Here's how the part is built. I have some questions about the finished solid (model axes, mm). Face numbers are marked on the shaded views. A direction names the side the tool comes from. Round coordinates to 2 decimals unless told otherwise and drop trailing zeros. Write each loop counter-clockwise with the first axis right and the second up, starting at its lowest first coordinate (ties: lowest second). Pieces come first, ordered by that corner, then holes. Notation, with made-up numbers: (17.25, 31.25) - (28.25, 31.25) arc R31 ccw to (28.25, 61.25) - close; hole circle Ø8 at (41.5, -23.75). An arc over 180 degrees is marked (long way). One line per question, with ' | ' between items. Start each with the question number.
(1) Will these pins go through, and if not, where does the flat tip stop? pin 1 (11 mm diameter, centred on x = -95.5, y = -3.5, fed in from +Z); pin 2 (1.6 mm diameter, centred on y = -43.5, z = -120.5, fed in from +X); pin 3 (1 mm diameter, centred on y = -36, z = -56.5, fed in from -X).
(2) Imagine slicing it at C-C (y = -13.5). Write out the boundary of the cut face in (x, z).
(3) For the marked faces 1 and 2, which set-ups out of +Z, -Z, +X, -X, +Y, -Y let a thin tool reach every point of the face, with its end or its side?
(4) If I drill on L1, parallel to X at y = -44, z = -79; L2, parallel to X at y = -31, z = -190; L3, parallel to Y at x = -59.5, z = -171.5, over which ranges is the centre line in solid material (lowest first)?
(5) Imagine slicing it at D-D (x = -29). Write out the boundary of the cut face in (y, z).
(6) Imagine slicing it at A-A (x = -93). Write out the boundary of the cut face in (y, z).
(7) Thinking about a two-plate mould opening in X: for the marked faces 3 and 4, which applies, pulls with the +X half, pulls with the -X half, needs draft (parallel to the pull), parting line crosses it, or undercut?
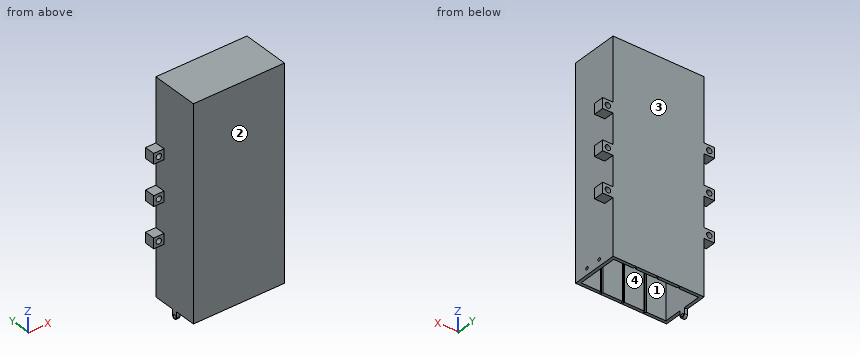
from build123d import *

# Parameters (mm, degrees)
SKETCH1_W           = 88
SKETCH1_H           = 46
SKETCH1_W_2         = 82
SKETCH1_H_2         = 40
BOSS_EXTRUDE1_DEPTH = 3
SKETCH3_W           = 88
SKETCH3_H           = 46
BOSS_EXTRUDE2_DEPTH = 200
SKETCH4_W           = 10
SKETCH4_H           = 10
BOSS_EXTRUDE3_DEPTH = 10
SKETCH7_R           = 2.6
CUT_EXTRUDE1_DEPTH  = 228.420315715
SKETCH8_W           = 3
SKETCH8_H           = 5
BOSS_EXTRUDE4_DEPTH = 8
FILLET1_RADIUS      = 2.5
FILLET1_LENGTH      = 3
SKETCH10_R          = 1.5
CUT_EXTRUDE3_DEPTH  = 10
SKETCH9_R           = 1.5
CUT_EXTRUDE4_DEPTH  = 10


with BuildPart() as part:
    # Sketch1 → Boss-Extrude1 (new body)
    # profile 1 of 2: a face of its own
    with BuildSketch(Plane.XY):
        with Locations((-44, -23)):
            Rectangle(SKETCH1_W, SKETCH1_H)
        with Locations((-44, -23)):
            Rectangle(SKETCH1_W_2, SKETCH1_H_2, mode=Mode.SUBTRACT)
    # profile 2 of 2: a face of its own
    with BuildSketch(Plane.XY):
        with Locations((-44, -23)):
            Rectangle(SKETCH1_W_2, SKETCH1_H_2)
    extrude(amount=BOSS_EXTRUDE1_DEPTH)

    # Sketch3 → Boss-Extrude2 (add)
    with BuildSketch(Plane(origin=(0, 0, 0), x_dir=(-1, 0, 0), z_dir=(0, 0, -1))):
        with Locations((44, -23)):
            Rectangle(SKETCH3_W, SKETCH3_H)
        Polygon((24, -3), (43, -3), (43, -1.5), (45, -1.5), (45, -3), (64, -3), (64, -1.5), (66, -1.5), (66, -3), (85, -3), (85, -43), (66, -43), (66, -44.5), (64, -44.5), (64, -43), (45, -43), (45, -44.5), (43, -44.5), (43, -43), (24, -43), (24, -44.5), (22, -44.5), (22, -43), (3, -43), (3, -3), (22, -3), (22, -1.5), (24, -1.5), align=None, mode=Mode.SUBTRACT)
    extrude(amount=BOSS_EXTRUDE2_DEPTH)

    # Sketch4 → Boss-Extrude3 (add)
    with BuildSketch(Plane(origin=(0, 0, 0), x_dir=(1, 0, 0), z_dir=(0, 1, 0))):
        with Locations((5, 141)):
            Rectangle(SKETCH4_W, SKETCH4_H)
        with Locations((5, 102)):
            Rectangle(SKETCH4_W, SKETCH4_H)
        with Locations((5, 63)):
            Rectangle(SKETCH4_W, SKETCH4_H)
        with Locations((-93, 141)):
            Rectangle(SKETCH4_W, SKETCH4_H)
        with Locations((-93, 102)):
            Rectangle(SKETCH4_W, SKETCH4_H)
        with Locations((-93, 63)):
            Rectangle(SKETCH4_W, SKETCH4_H)
    extrude(amount=-BOSS_EXTRUDE3_DEPTH)

    # Sketch7 → Cut-Extrude1 (cut, through all)
    with BuildSketch(Plane(origin=(0, 0, 0), x_dir=(1, 0, 0), z_dir=(0, 1, 0))):
        with Locations(Location((-93, 141, 0), (0, 0, 270))):
            Circle(SKETCH7_R)
        with Locations(Location((-93, 102, 0), (0, 0, 270))):
            Circle(SKETCH7_R)
        with Locations(Location((-93, 63, 0), (0, 0, 270))):
            Circle(SKETCH7_R)
        with Locations(Location((5, 141, 0), (0, 0, 270))):
            Circle(SKETCH7_R)
        with Locations(Location((5, 102, 0), (0, 0, 270))):
            Circle(SKETCH7_R)
        with Locations(Location((5, 63, 0), (0, 0, 270))):
            Circle(SKETCH7_R)
    extrude(amount=-CUT_EXTRUDE1_DEPTH, mode=Mode.SUBTRACT)

    # Sketch8 → Boss-Extrude4 (add)
    with BuildSketch(Plane(origin=(0, 0, -200), x_dir=(-1, 0, 0), z_dir=(0, 0, -1))):
        with Locations((86.5, -23)):
            Rectangle(SKETCH8_W, SKETCH8_H)
    extrude(amount=BOSS_EXTRUDE4_DEPTH)

    # Fillet1: full round fillet: the end face becomes a half cylinder, R = half its width
    fillet1_face = Plane((-86.5, -23, -208), x_dir=(-1, 0, 0), z_dir=(0, 0, -1))  # on the end face: x along it, z out of the body
    fillet1_slab = fillet1_face.offset(-FILLET1_RADIUS / 2) * Box(FILLET1_LENGTH, 2 * FILLET1_RADIUS, FILLET1_RADIUS, mode=Mode.PRIVATE)  # the body's end, R deep
    fillet1_round = Plane((-86.5, -23, -205.5), x_dir=(0, 0, -1), z_dir=(-1, 0, 0)) * Cylinder(FILLET1_RADIUS, FILLET1_LENGTH, mode=Mode.PRIVATE)  # its axis R under the face
    add(fillet1_slab - fillet1_round, mode=Mode.SUBTRACT)

    # Sketch10 → Cut-Extrude3 (cut)
    with BuildSketch(Plane(origin=(0, 0, 0), x_dir=(0, 0, -1), z_dir=(1, 0, 0))):
        with Locations(Location((193.8, -32, 0), (0, 0, 90))):
            Circle(SKETCH10_R)
        with Locations(Location((193.8, -17, 0), (0, 0, 90))):
            Circle(SKETCH10_R)
    extrude(amount=-CUT_EXTRUDE3_DEPTH, mode=Mode.SUBTRACT)

    # Sketch9 → Cut-Extrude4 (cut)
    with BuildSketch(Plane.ZY.offset(88)):
        with Locations((-205.5, -23)):
            Circle(SKETCH9_R)
    extrude(amount=-CUT_EXTRUDE4_DEPTH, mode=Mode.SUBTRACT)


solid = part.part
Check sheet entries:
1) pin 1: z = -58 | pin 2: x = 0 | pin 3: x = -88
2) outline: (-88, -200) - (-85, -200) - (-85, 0) - (-3, 0) - (-3, -200) - (0, -200) - (0, 3) - (-88, 3) - close
3) face 1: -Z | face 2: +Z, -Z, +X, -X, -Y
4) L1: -88 to -66, -64 to -45, -43 to -24, -22 to 0 | L2: -88 to -85, -3 to 0 | L3: -46 to -43, -3 to 0
5) outline: (-46, -200) - (-43, -200) - (-43, 0) - (-3, 0) - (-3, -200) - (0, -200) - (0, 3) - (-46, 3) - close
6) outline: (-10, -146) - (0, -146) - (0, -143.6) - (-10, -143.6) - close; (-10, -138.4) - (0, -138.4) - (0, -136) - (-10, -136) - close; (-10, -107) - (0, -107) - (0, -104.6) - (-10, -104.6) - close; (-10, -99.4) - (0, -99.4) - (0, -97) - (-10, -97) - close; (-10, -68) - (0, -68) - (0, -65.6) - (-10, -65.6) - close; (-10, -60.4) - (0, -60.4) - (0, -58) - (-10, -58) - close
7) face 3: needs draft | face 4: undercut
